Check sheet for the drawn part. Datum: minimum x, y, z corner. Units: mm. A direction names the side the tool comes from. Give positions to 0.01 mm unless a question says otherwise; leave off trailing zeros. Loops run counter-clockwise (first coordinate to the right, second up) from the corner with the lowest first, then second, coordinate; pieces in that order, holes last. Notation, with made-up numbers: (32.25, 85) - (46.25, 85) arc R34 cw to (46.25, 116) - close; hole circle Ø1 at (-22.75, 34.25). An arc over 180 degrees is marked (long way). Answer in a Markdown table with one row per item.
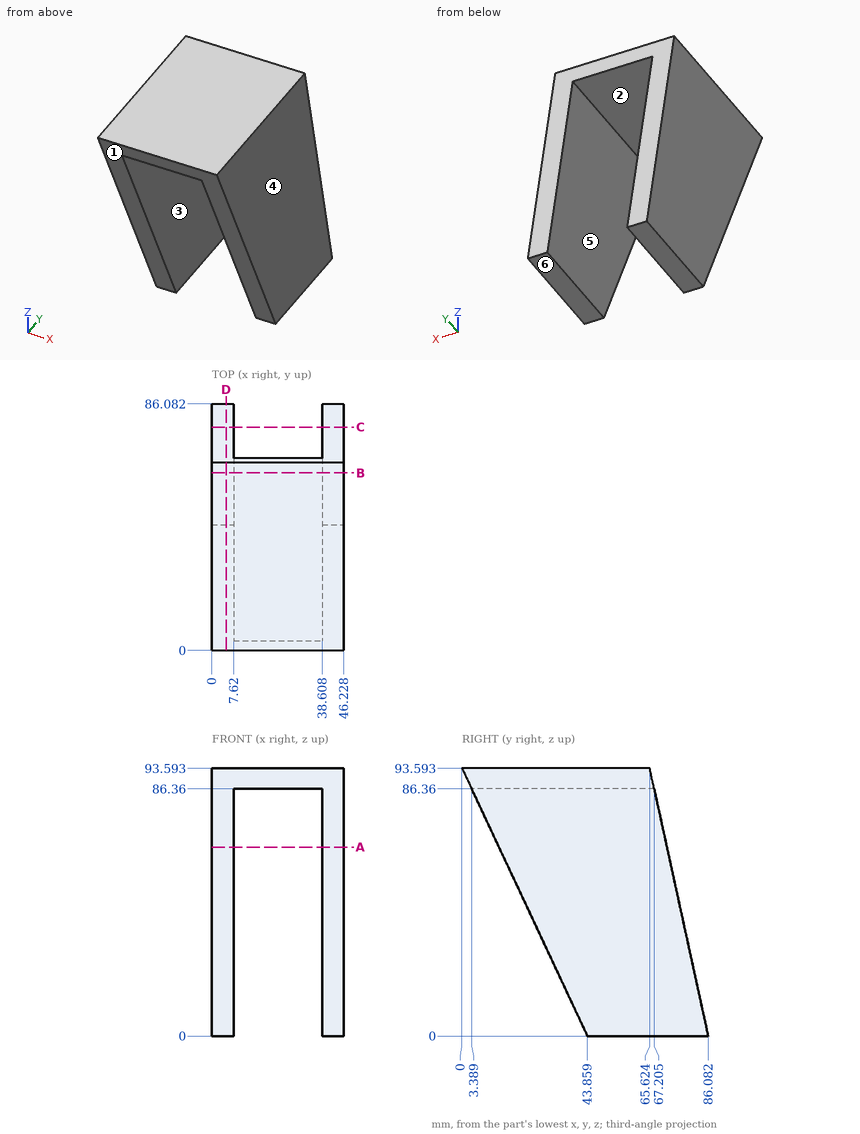
Q1. Tool access check on the marked faces 5 and 6. Record the directions out of +Z, -Z, +X, -X, +Y, -Y that give a thin tool (end or side, any length) a straight path to the whole face; none if there is none.
Completed:
| item | result |
|---|---|
| face 5 | -Z, +Y, -Y |
| face 6 | -Z, +X, -X, +Y, -Y |
Q2. Sectioned sample at B-B (y = 62). Record the cut outline in (x, z).
Completed:
| item | result |
|---|---|
| outline | (0, 0) - (7.62, 0) - (7.62, 86.36) - (38.61, 86.36) - (38.61, 0) - (46.23, 0) - (46.23, 93.59) - (0, 93.59) - close |
Q3. Sectioned sample at C-C (y = 78). Record the cut outline in (x, z).
Completed:
| item | result |
|---|---|
| outline | (0, 0) - (7.62, 0) - (7.62, 36.97) - (0, 36.97) - close; (38.61, 0) - (46.23, 0) - (46.23, 36.97) - (38.61, 36.97) - close |
Q4. Go/stop test with flat-tipped pins: P1, Ø15.5, axis at x = 19, y = 46.5, coming from the -Z side; P2, Ø3, axis at x = 38.5, z = 17, coming from the -Y side. Record where each tip stops, or that it passes through.
Completed:
| item | result |
|---|---|
| P1 | z = 86.36 |
| P2 | y = 35.19 |
Q5. Draft check along X on the marked faces 1, 2, 3 and 4. Enter one of: +X half, -X half, draft (parallel to the pull), parting line (faces both ways), or undercut.
Completed:
| item | result |
|---|---|
| face 1 | draft |
| face 2 | undercut |
| face 3 | undercut |
| face 4 | +X half |
Q6. Sectioned sample at D-D (x = 5). Record the cut outline in (y, z) (1 decimal), and give its area (3 significant figures).
Completed:
| item | result |
|---|---|
| outline | (0, 93.6) - (43.9, 0) - (86.1, 0) - (65.6, 93.6) - close |
| area | 5,050 mm^2 |
Q7. Thickness scan on line 1 (X direction, y = 33, z = 82.5); line 2 (Z direction, x = 21.5, y = 40); line 3 (Y direction, x = 39, z = 37.5) (1 decimal). Record the ranges inside material, lowest first.
Completed:
| item | result |
|---|---|
| line 1 | 0 to 7.62, 38.61 to 46.23 |
| line 2 | 86.36 to 93.59 |
| line 3 | 26.3 to 77.9 |
Q8. Sectioned sample at A-A (z = 66). Record the cut outline in (x, y) (1 decimal).
Completed:
| item | result |
|---|---|
| outline | (0, 12.9) - (7.6, 12.9) - (7.6, 71.7) - (0, 71.7) - close; (38.6, 12.9) - (46.2, 12.9) - (46.2, 71.7) - (38.6, 71.7) - close |
